Could you check a few things on this model? Use its own coordinates, in mm. A direction names the side the tool comes from. Coordinates: 2 decimals unless noted, no trailing zeros. Write each loop counter-clockwise with the first axis right and the second up, starting at its lowest first coordinate (ties: lowest second). Pieces come first, ordered by that corner, then holes.
Item 1: If I drill on probe 1 along X at (y, z) = (0.85, 0); probe 2 along X at (y, z) = (8, 0); probe 3 along Y at (x, z) = (0, 3.6), over which ranges is the centre line in solid material (lowest first)?
Item 2: Thinking about a two-plate mould opening in Z: for faces 1 (the cylindrical face through (14.531, 1.479, -15.846)), 2 (the flat face through (0, 3, 0)), 3 (the flat face through (0, 0, 0)), which applies, +Z half, -Z half, draft (parallel to the pull), parting line (faces both ways), or undercut?
Item 3: For P1, Ø12, axis at x = 5, z = 5.5, coming from the +Y side; P2, Ø1, axis at y = 2, z = 14, coming from the +X side; P3, Ø1.4, axis at x = 0, z = -12, coming from the +Y side; P4, Ø5, axis at y = 4.5, z = 11.5, coming from the -X side, each with a flat end and sliding along its axis, tell me the tip position at first contact or that it passes through.
Item 4: I want a section at A-A on z = 0. Please give me the cut outline in (x, y), then the cut area to 3 significant figures.
Item 5: Which directions (+Z, -Z, +X, -X, +Y, -Y) give clear straight access to the entire face, cutting with the end or side of a thin tool? Please do faces 4 (the cylindrical face through (-1.168, 7.93, 2.817)), 5 (the cylindrical face through (-1.05, 7.15, 3.72)).
Item 6: I want a section at B-B on y = 2. Please give me the cut outline in (x, z), then the cut area to 3 significant figures.
Item 7: I want a section at C-C on x = 0. State how many separate pieces and enclosed holes the cut face has, then the cut area to 3 significant figures.
Item 8: I want a section at D-D on z = -12. Please give me the cut outline in (x, y).
from build123d import *

# Parameters (mm, degrees)
SKETCH_1_R               = 21.5
EXTRUDE_1_DEPTH          = 3
SKETCH_2_R               = 4.55
SKETCH_2_R_2             = 3.05
EXTRUDE_2_DEPTH          = 10
SKETCH_3_R               = 1.05
CUT_EXTRUDE_1_DEPTH      = 8.5
CUT_EXTRUDE_2_REACH      = 34.008
SKETCH_4_R               = 1.2
PATTERN_CIRCULAR_1_COUNT = 4
FILLET_1_R               = 1


with BuildPart() as part:
    # 草图1 → 凸台-拉伸1 (new body)
    with BuildSketch(Plane(origin=(0, 0, 0), x_dir=(1, 0, 0), z_dir=(0, 1, 0))):
        with Locations(Location((0, 0, 0), (0, 0, 270))):
            Circle(SKETCH_1_R)
    extrude(amount=EXTRUDE_1_DEPTH)

    # 草图2 → 凸台-拉伸2 (add)
    with BuildSketch(Plane(origin=(0, 3, 0), x_dir=(1, 0, 0), z_dir=(0, 1, 0))):
        with Locations(Location((0, 0, 0), (0, 0, 270))):
            Circle(SKETCH_2_R)
        with Locations(Location((0, 0, 0), (0, 0, 270))):
            Circle(SKETCH_2_R_2, mode=Mode.SUBTRACT)
    extrude(amount=EXTRUDE_2_DEPTH)

    # 草图3 → 切除-拉伸1 (cut, symmetric)
    with BuildSketch(Plane.XY):
        with Locations((0, 7.1)):
            Circle(SKETCH_3_R)
    extrude(amount=CUT_EXTRUDE_1_DEPTH, both=True, mode=Mode.SUBTRACT)

    # 草图4 → 切除-拉伸2 (cut, up to next)
    with BuildSketch(Plane(origin=(0, 3, 0), x_dir=(1, 0, 0), z_dir=(0, 1, 0)), mode=Mode.PRIVATE) as cut_extrude_2_sk1:
        with Locations(Location((12, 0, 0), (0, 0, 270))):
            Circle(SKETCH_4_R)
    cut_extrude_2_tool1 = extrude(cut_extrude_2_sk1.sketch, amount=-CUT_EXTRUDE_2_REACH, mode=Mode.PRIVATE) & part.part
    cut_extrude_2 = cut_extrude_2_tool1.solids().sort_by_distance((12, 3, 0))[0]
    add(cut_extrude_2, mode=Mode.SUBTRACT)

    # 阵列(圆周)1: 切除-拉伸2 ×4 about axis
    pattern_circular_1_axis = Axis((0, 0, 0), (0, 1, 0))
    for i in range(1, PATTERN_CIRCULAR_1_COUNT):
        add(cut_extrude_2.rotate(pattern_circular_1_axis, i * 360 / PATTERN_CIRCULAR_1_COUNT), mode=Mode.SUBTRACT)

    # 圆角1
    fillet_1_edges = [part.edges().sort_by_distance(p)[0] for p in [
        (0, 3, -4.55),
    ]]
    fillet(fillet_1_edges, radius=FILLET_1_R)


solid = part.part
Response values:
1. probe 1: x = -21.5 to -13.2, -10.8 to 10.8, 13.2 to 21.5
1. probe 2: x = -4.55 to -3.05, 3.05 to 4.55
1. probe 3: y = 0 to 6.05, 8.15 to 13
2. face 1: parting line
2. face 2: undercut
2. face 3: draft
3. P1: stops at y = 13
3. P2: stops at x = 16.73
3. P3: passes through
3. P4: stops at x = -19.29
4. outline: (-21.5, 0) - (-13.2, 0) - (-13.2, 3) - (-21.5, 3) - close; (-10.8, 0) - (10.8, 0) - (10.8, 3) - (5.55, 3) arc R1 cw to (4.55, 4) - (4.55, 13) - (3.05, 13) - (3.05, 3) - (-3.05, 3) - (-3.05, 13) - (-4.55, 13) - (-4.55, 4) arc R1 cw to (-5.55, 3) - (-10.8, 3) - close; (13.2, 0) - (21.5, 0) - (21.5, 3) - (13.2, 3) - close
4. area: 145 mm2
5. face 4: +Y
5. face 5: +Z, -Z
6. outline: circle Ø43 at (0, 0); hole circle Ø2.4 at (-12, 0); hole circle Ø2.4 at (0, -12); hole circle Ø2.4 at (0, 12); hole circle Ø2.4 at (12, 0)
6. area: 1,430 mm2
7. separate pieces: 5
7. enclosed holes: 0
7. area: 139 mm2
8. outline: (-17.84, 0) - (-1.2, 0) - (-1.2, 3) - (-17.84, 3) - close; (1.2, 0) - (17.84, 0) - (17.84, 3) - (1.2, 3) - close
